from build123d import *

# Parameters (mm, degrees)
SKETCH2_W                       = 9.525
SKETCH2_H                       = 63.5
BOSS_EXTRUDE1_DEPTH             = 22.225
BOSS_EXTRUDE1_2_DEPTH           = 22.225
BOSS_EXTRUDE3_REACH             = 69.295
SKETCH3_R                       = 9.525
SKETCH4_R                       = 9.525
BOSS_EXTRUDE4_DEPTH             = 74.6125
F_43_0_089_DIAMETER_HOLE1_D     = 2.2606
F_43_0_089_DIAMETER_HOLE1_DEPTH = 6.35
F_43_0_089_DIAMETER_HOLE1_TIP   = 0.679152758


with BuildPart() as part:
    # Sketch2 → Boss-Extrude1 (new body)
    with BuildSketch(Plane.XY):
        with Locations((-19.05, 19.074189237)):
            Rectangle(SKETCH2_W, SKETCH2_H)
    extrude(amount=BOSS_EXTRUDE1_DEPTH)


with BuildPart() as body_2:
    # Sketch2 → Boss-Extrude1 2 (new body)
    with BuildSketch(Plane.XY):
        with Locations((19.05, 19.074189237)):
            Rectangle(SKETCH2_W, SKETCH2_H)
    extrude(amount=BOSS_EXTRUDE1_2_DEPTH)

    # Sketch3 → Boss-Extrude3 (add, up to next)
    with BuildSketch(Plane(origin=(-14.2875, 0, 0), x_dir=(0, 0, -1), z_dir=(1, 0, 0)), mode=Mode.PRIVATE) as boss_extrude3_sk1:
        with Locations(Location((-11.1125, 34.949189237, 0), (0, 0, 270))):
            Circle(SKETCH3_R)
    boss_extrude3_tool1 = extrude(boss_extrude3_sk1.sketch, amount=BOSS_EXTRUDE3_REACH, mode=Mode.PRIVATE) - body_2.part

    add(part.part)  # Boss-Extrude3 merges part
    add(boss_extrude3_tool1.solids().sort_by_distance((-14.2875, 34.949189, 11.1125))[0])

    # Sketch4 → Boss-Extrude4 (add)
    with BuildSketch(Plane(origin=(23.8125, 0, 0), x_dir=(0, 0, -1), z_dir=(1, 0, 0))):
        with Locations(Location((-11.1125, 3.199189237, 0), (0, 0, 270))):
            Circle(SKETCH4_R)
    boss_extrude4 = extrude(amount=BOSS_EXTRUDE4_DEPTH)

    # Mirror1: Boss-Extrude4 across plane
    add(boss_extrude4.mirror(Plane(origin=(0, 0, 0), x_dir=(0, 0, 1), z_dir=(1, 0, 0))))

    # #43 (0.089) Diameter Hole1
    with Locations(Plane(origin=(23.8125, 0, 0), x_dir=(0, 0, -1), z_dir=(1, 0, 0))):
        with Locations((-17.4625, 14.311689237), (-4.7625, 14.311689237)):
            Hole(F_43_0_089_DIAMETER_HOLE1_D / 2, depth=F_43_0_089_DIAMETER_HOLE1_DEPTH)
            with Locations((0, 0, -(F_43_0_089_DIAMETER_HOLE1_DEPTH + F_43_0_089_DIAMETER_HOLE1_TIP / 2))):  # 118° drill point
                Cone(0, F_43_0_089_DIAMETER_HOLE1_D / 2, F_43_0_089_DIAMETER_HOLE1_TIP, mode=Mode.SUBTRACT)


solid = body_2.part
Work out the finished part from the listing and answer in its coordinate system (mm). A direction names the side the tool comes from. Round coordinates to 2 decimals unless told otherwise and drop trailing zeros. Write each loop counter-clockwise with the first axis right and the second up, starting at its lowest first coordinate (ties: lowest second). Pieces come first, ordered by that corner, then holes. Notation, with made-up numbers: M 87.25,17.25 L 100.25,17.25 A6 cw 100.25,24.25 Z; hole C 53.5,84 d11. An arc over 180 degrees is marked long. Use a Markdown table: item, result.
1) The part is cut by section C-C on z = 14.5. Give the vertices of the cut face in (x, y) (1 decimal), plus the area to 3 significant figures.
Taken from the geometry:
| item | result |
|---|---|
| outline | M -98.4,-5.7 L -23.8,-5.7 L -23.8,-12.7 L -14.3,-12.7 L -14.3,26 L 14.3,26 L 14.3,-12.7 L 23.8,-12.7 L 23.8,-5.7 L 98.4,-5.7 L 98.4,12.1 L 23.8,12.1 L 23.8,50.8 L 14.3,50.8 L 14.3,43.9 L -14.3,43.9 L -14.3,50.8 L -23.8,50.8 L -23.8,12.1 L -98.4,12.1 Z |
| area | 4,380 mm2 |
2) The part is cut by section B-B on y = 39. Give the vertices of the cut face in (x, z) (1 decimal).
Taken from the geometry:
| item | result |
|---|---|
| outline | M -23.8,0 L -14.3,0 L -14.3,2.5 L 14.3,2.5 L 14.3,0 L 23.8,0 L 23.8,22.2 L 14.3,22.2 L 14.3,19.7 L -14.3,19.7 L -14.3,22.2 L -23.8,22.2 Z |
3) The part is cut by section D-D on y = -0.5. Give the vertices of the cut face in (x, z) (1 decimal).
Taken from the geometry:
| item | result |
|---|---|
| outline | M -98.4,2.3 L -23.8,2.3 L -23.8,0 L -14.3,0 L -14.3,22.2 L -23.8,22.2 L -23.8,19.9 L -98.4,19.9 Z; M 14.3,0 L 23.8,0 L 23.8,2.3 L 98.4,2.3 L 98.4,19.9 L 23.8,19.9 L 23.8,22.2 L 14.3,22.2 Z |
4) The part is cut by section A-A on y = 8. Give the vertices of the cut face in (x, z) (1 decimal).
Taken from the geometry:
| item | result |
|---|---|
| outline | M -98.4,2.9 L -23.8,2.9 L -23.8,0 L -14.3,0 L -14.3,22.2 L -23.8,22.2 L -23.8,19.3 L -98.4,19.3 Z; M 14.3,0 L 23.8,0 L 23.8,2.9 L 98.4,2.9 L 98.4,19.3 L 23.8,19.3 L 23.8,22.2 L 14.3,22.2 Z |
5) Consider line 1 (X direction, y = -6, z = 11.25) (1 decimal); line 2 (X direction, y = 43, z = 17.5); line 3 (X direction, y = 42, z = 11). Determine where each line is inside the solid, lowest interval first. Write a range as [from, to].
Taken from the geometry:
| item | result |
|---|---|
| line 1 | x = [-98.4, -14.3], [14.3, 98.4] |
| line 2 | x = [-23.81, -14.29], [14.29, 23.81] |
| line 3 | x = [-23.81, 23.81] |
6) Determine the mould class of faces 6 (the face through (-14.288, 12, 11)), 7 (the face through (19, 20, 0)), 8 (the face through (-23.812, 26, 11)) for opening direction X: pulls with the +X half, pulls with the -X half, needs draft (parallel to the pull), parting line crosses it, or undercut.
Taken from the geometry:
| item | result |
|---|---|
| face 6 | undercut |
| face 7 | needs draft |
| face 8 | pulls with the -X half |
7) Which of the six approach directions +Z, -Z, +X, -X, +Y, -Y give full straight-line access (tool end or side, diameter ignored) to faces 1 (the face through (-98.425, 3, 11)), 2 (the face through (60.6, -5.9, 8.3)), 3 (the face through (-60.6, -5.9, 8.3)), 4 (the face through (-0.2, 42.508, 16.908)), 5 (the face through (-19, 50.824, 11))?
Taken from the geometry:
| item | result |
|---|---|
| face 1 | +Z, -Z, -X, +Y, -Y |
| face 2 | +X |
| face 3 | -X |
| face 4 | none |
| face 5 | +Z, -Z, +X, -X, +Y |
8) Flat-ended cylindrical pins translate along their axes: pin 1 (11 mm diameter, centred on y = 32, z = 7.5, fed in from +X); pin 2 (8 mm diameter, centred on x = -41, y = 18.5, fed in from -Z); pin 3 (3 mm diameter, centred on y = 14.31, z = 4.76, fed in from -X); pin 4 (1 mm diameter, centred on x = 60.5, z = 10, fed in from -Y). Find the tip coordinate at first contact, or state that the pin passes through.
Taken from the geometry:
| item | result |
|---|---|
| pin 1 | stops at x = 23.81 |
| pin 2 | passes through |
| pin 3 | stops at x = -23.81 |
| pin 4 | stops at y = -6.31 |
